Verification items for the finished model (mm, model axes). Face numbers are marked on the shaded views. A direction names the side the tool comes from. Coordinates: 2 decimals unless noted, no trailing zeros. Write each loop counter-clockwise with the first axis right and the second up, starting at its lowest first coordinate (ties: lowest second). Pieces come first, ordered by that corner, then holes. Notation, with made-up numbers: M 10.25,38.25 L 40.25,38.25 A10 cw 40.25,43.25 Z; hole C 27,37.5 d9. An arc over 180 degrees is marked long. Answer in a Markdown table with one row per item.
from build123d import *

# Parameters (mm, degrees)
F0_R     = 3.175
F1_DEPTH = 6.35
F2_DEPTH = 9.525
F3_R     = 3.175
F4_DEPTH = 12.7


with BuildPart() as f1:
    # F0 (on Front) → F1 (new body, symmetric)
    with BuildSketch(Plane.XZ):
        with BuildLine():
            ThreePointArc((8.975765, -6.223), (10.424092, -3.260121), (10.922, 0))
            ThreePointArc((10.922, 0), (-3.260121, 10.424092), (-8.975765, -6.223))
            Line((-8.975765, -6.223), (8.975765, -6.223))
        make_face()
        Circle(F0_R, mode=Mode.SUBTRACT)
    extrude(amount=F1_DEPTH, both=True)

    # F0 (on Front) → F2 (join, symmetric)
    with BuildSketch(Plane.XZ):
        Circle(F0_R)
    extrude(amount=F2_DEPTH, both=True)

    # F3 (on face) → F4 (cut)
    with BuildSketch(Plane(origin=(0, 0, -6.223), x_dir=(1, 0, 0), z_dir=(0, 0, -1))):
        Circle(F3_R)
    extrude(amount=-F4_DEPTH, mode=Mode.SUBTRACT)


solid = f1.part
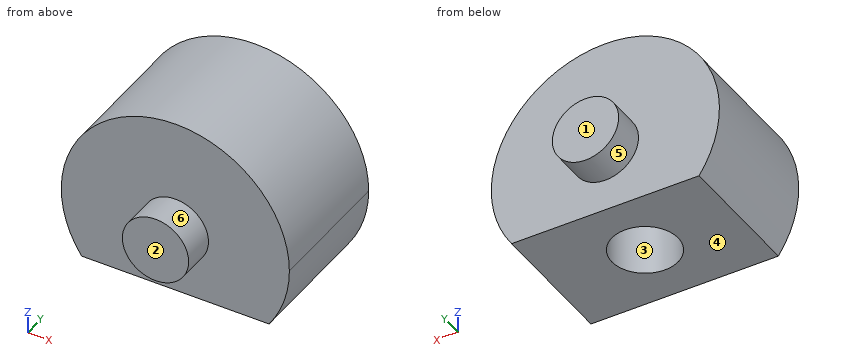
1) Thickness scan on L1, parallel to Y at x = 0, z = 4 (3 decimals); L2, parallel to Y at x = 7, z = 2.5; L3, parallel to X at y = 0, z = -0.25 (3 decimals). Record the ranges inside material, lowest first. Write a range as [from, to].
Response values:
| item | result |
|---|---|
| L1 | y = [-6.35, -3.175], [3.175, 6.35] |
| L2 | y = [-6.35, 6.35] |
| L3 | x = [-10.919, -3.175], [3.175, 10.919] |
2) Sectioned sample at A-A (z = 2). Record the cut outline in (x, y) (3 decimals).
Response values:
| item | result |
|---|---|
| outline | M -10.737,-6.35 L -2.466,-6.35 L -2.466,-9.525 L 2.466,-9.525 L 2.466,-6.35 L 10.737,-6.35 L 10.737,6.35 L 2.466,6.35 L 2.466,9.525 L -2.466,9.525 L -2.466,6.35 L -10.737,6.35 Z; hole C 0,0 d6.35 |
3) Depth check by flat-ended pin: pin 1 (6 mm diameter, centred on x = 8, y = -0.5, fed in from +Z); pin 2 (8 mm diameter, centred on y = 6, z = 9, fed in from -X); pin 3 (5 mm diameter, centred on x = 3.5, y = -7.5, fed in from +Z); pin 4 (10 mm diameter, centred on x = 4, z = 3, fed in from -Y) (3 decimals). Enter the tip coordinate at first touch or a pass-through.
Response values:
| item | result |
|---|---|
| pin 1 | stops at z = 9.71 |
| pin 2 | stops at x = -9.71 |
| pin 3 | stops at z = 10.85 |
| pin 4 | stops at y = -9.525 |
4) Sectioned sample at B-B (x = 0). Record the cut outline in (y, z) (3 decimals), then the cut area to 3 significant figures.
Response values:
| item | result |
|---|---|
| outline | M -9.525,-3.175 L -6.35,-3.175 L -6.35,-6.223 L -3.175,-6.223 L -3.175,6.477 L 3.175,6.477 L 3.175,-6.223 L 6.35,-6.223 L 6.35,-3.175 L 9.525,-3.175 L 9.525,3.175 L 6.35,3.175 L 6.35,10.922 L -6.35,10.922 L -6.35,3.175 L -9.525,3.175 Z |
| area | 177 mm² |
5) Sectioned sample at C-C (y = 0). Record the cut outline in (x, z) (3 decimals), then the cut area to 3 significant figures.
Response values:
| item | result |
|---|---|
| outline | M -8.976,-6.223 L -3.175,-6.223 L -3.175,6.477 L 3.175,6.477 L 3.175,-6.223 L 8.976,-6.223 A10.922 ccw 10.922,0 A10.922 ccw long Z |
| area | 235 mm² |
6) Release check for a two-part mould opening along Y. For the marked faces 1, 2, 3 and 4 record: +Y half, -Y half, draft (parallel to the pull), parting line (faces both ways), or undercut.
Response values:
| item | result |
|---|---|
| face 1 | +Y half |
| face 2 | -Y half |
| face 3 | undercut |
| face 4 | draft |
7) Sectioned sample at D-D (z = -2.5). Record the cut outline in (x, y) (3 decimals).
Response values:
| item | result |
|---|---|
| outline | M -10.632,-6.35 L -1.957,-6.35 L -1.957,-9.525 L 1.957,-9.525 L 1.957,-6.35 L 10.632,-6.35 L 10.632,6.35 L 1.957,6.35 L 1.957,9.525 L -1.957,9.525 L -1.957,6.35 L -10.632,6.35 Z; hole C 0,0 d6.35 |
8) Tool access check on the marked faces 5 and 6. Record the directions out of +Z, -Z, +X, -X, +Y, -Y that give a thin tool (end or side, any length) a straight path to the whole face; none if there is none.
Response values:
| item | result |
|---|---|
| face 5 | +Y |
| face 6 | -Y |
